Answer from the drawing. Dimensions are ordinates in mm from the lowest x, y and z of the part. Give positions to 0.01 mm unless a question says otherwise; leave off trailing zeros. Write each loop counter-clockwise with the first axis right and the second up, starting at its lowest first coordinate (ties: lowest second). Pieces come first, ordered by that corner, then holes.
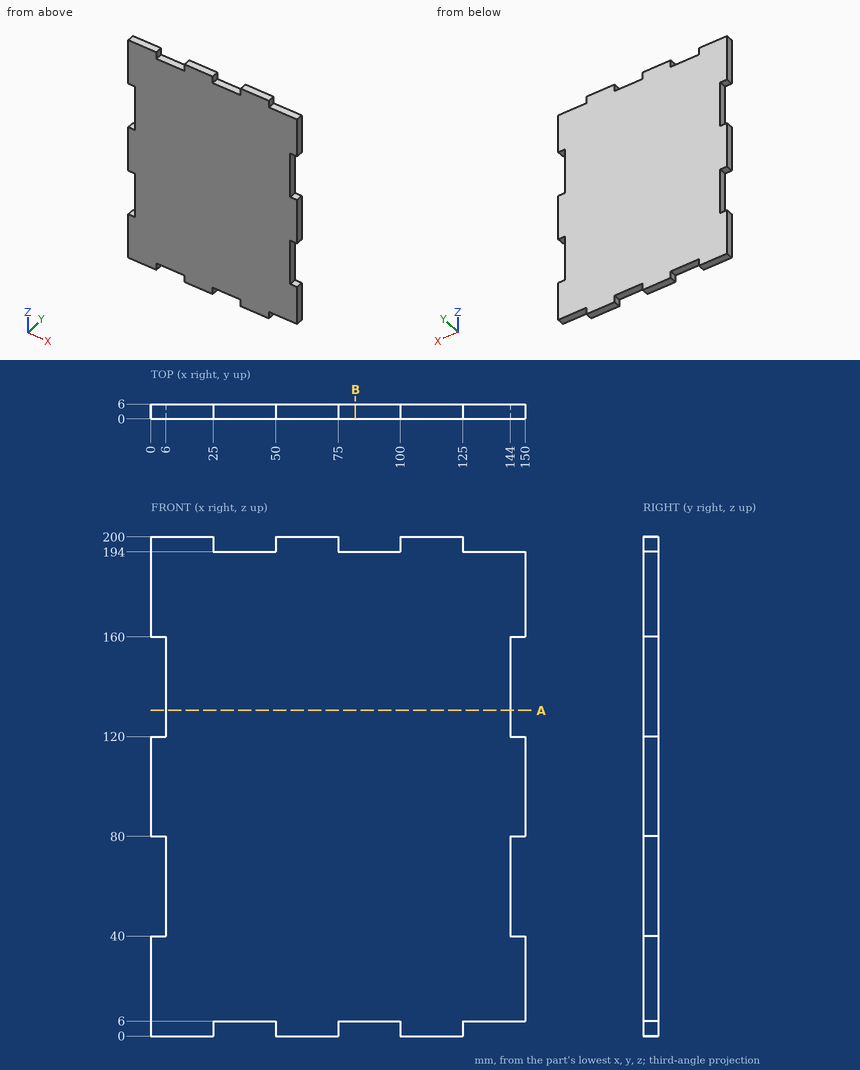
Item 1: A cutting plane is placed at B-B, the plane x = 82. Give the vertices of the cut face in (y, z), plus the area to 3 significant figures.
Conclusion:
outline: (0, 6) - (6, 6) - (6, 194) - (0, 194) - close
area: 1,130 mm2
Item 2: Consider probe 1 along X at (y, z) = (5.5, 47.5); probe 2 along Z at (x, y) = (81, 3.5). Determine where each line is inside the solid, lowest interval first.
Conclusion:
probe 1: x = 6 to 144
probe 2: z = 6 to 194
Item 3: Each of these flat-tipped pins is pushed along its axis until it touches: P1, Ø3, axis at x = 92.5, y = 1.5, coming from the +Z side; P2, Ø1.8, axis at y = 3.5, z = 198.5, coming from the +X side; P3, Ø3, axis at x = 41, y = 3, coming from the -Z side. Where does it stop, or does it pass through?
Conclusion:
P1: stops at z = 194
P2: stops at x = 125
P3: stops at z = 6
Item 4: A cutting plane is placed at A-A, the plane z = 130.5. Give the vertices of the cut face in (x, y).
Conclusion:
outline: (6, 0) - (144, 0) - (144, 6) - (6, 6) - close
